Build history of the part. All positions in model axes, mm. Coordinates: 2 decimals unless noted, no trailing zeros. Loops run counter-clockwise (first coordinate to the right, second up) from the corner with the lowest first, then second, coordinate; pieces in that order, holes last. Notation, with made-up numbers: M 36.25,61.5 L 44.25,61.5 A32 cw 44.25,97.5 Z; hole C 8,33 d1. An arc over 180 degrees is marked long. Write each question's results on one line, items separated by ' | '. Start each with the question number.
from build123d import *

# Parameters (mm, degrees)
PRISM002_DEPTH           = 2.6
PRISM002_PLACEMENT_ANGLE = 45
ARRAY_COUNT              = 4
CYLINDER003_R            = 5.25
CYLINDER003_DEPTH        = 36
CYLINDER003_ROLL_ANGLE   = 90
SKETCH011_R              = 29
PAD006_DEPTH             = 16
SKETCH_R                 = 27.4
POCKET_DEPTH             = 1
SKETCH012_R              = 1.6
POCKET003_DEPTH          = 13
SKETCH013_W              = 16
SKETCH013_H              = 4
PAD_DEPTH                = 4
POCKET004_DEPTH          = 24
CHAMFER_SIZE             = 1


with BuildPart() as array:
    # Prism002 → Prism002 (new body)
    with BuildSketch(Plane.XY):
        Polygon((3.1, 0), (1.55, 2.684679), (-1.55, 2.684679), (-3.1, 0), (-1.55, -2.684679), (1.55, -2.684679), align=None)
    extrude(amount=PRISM002_DEPTH)


with BuildPart() as array_1:
    # Prism002 placement: moved
    add(array.part.moved(Location((-15.5563, 15.5563, 12.4))).rotate(Axis((-15.5563, 15.5563, 12.4), (0, 0, 1)), PRISM002_PLACEMENT_ANGLE))

    # Array: Array ×4 about axis
    array_axis = Axis((0, 0, 0), (0, 0, 1))


with BuildPart() as array_2:
    add(array_1.part)
    for i in range(1, ARRAY_COUNT):
        add(array_1.part.rotate(array_axis, i * 360 / ARRAY_COUNT))


with BuildPart() as laser_pointer:
    # Cylinder003 → Cylinder003 (new body)
    with BuildSketch(Plane.XY):
        Circle(CYLINDER003_R)
    extrude(amount=CYLINDER003_DEPTH)


with BuildPart() as laser_pointer_1:
    # Cylinder003 roll: moved
    add(laser_pointer.part.rotate(Axis((0, 0, 0), (1, 0, 0)), CYLINDER003_ROLL_ANGLE))


with BuildPart() as laser_pointer_2:
    # Cylinder003 placement: moved
    add(laser_pointer_1.part.moved(Location((0, 30, 8.5))))


with BuildPart() as laser_enclosure:
    # Sketch011 → Pad006 (new body)
    with BuildSketch(Plane.XY):
        Circle(SKETCH011_R)
    extrude(amount=PAD006_DEPTH)

    # Sketch → Pocket (cut)
    with BuildSketch(Plane.XY.offset(16)):
        Circle(SKETCH_R)
    extrude(amount=-POCKET_DEPTH, mode=Mode.SUBTRACT)

    # Sketch012 → Pocket003 (cut)
    with BuildSketch(Plane.XY.offset(15)):
        with Locations((-15.556349, 15.556349)):
            Circle(SKETCH012_R)
        with Locations((-15.556349, -15.556349)):
            Circle(SKETCH012_R)
        with Locations((15.556349, -15.556349)):
            Circle(SKETCH012_R)
        with Locations((15.556349, 15.556349)):
            Circle(SKETCH012_R)
        with BuildLine():
            ThreePointArc((-15.072779, -21.917375), (0, -26.6), (15.072779, -21.917375))
            Line((15.072779, -21.917375), (12.149548, -18.340897))
            ThreePointArc((18.340897, -12.149548), (12.445079, -12.445079), (12.149548, -18.340897))
            Line((21.91738, -15.072773), (18.340897, -12.149548))
            ThreePointArc((21.91738, -15.072773), (26.6, 4e-06), (21.917375, 15.072779))
            Line((21.917375, 15.072779), (18.340897, 12.149548))
            ThreePointArc((12.149548, 18.340897), (12.445079, 12.445079), (18.340897, 12.149548))
            Line((15.072779, 21.917375), (12.149548, 18.340897))
            ThreePointArc((15.072779, 21.917375), (0, 26.6), (-15.072779, 21.917375))
            Line((-15.072779, 21.917375), (-12.149548, 18.340897))
            ThreePointArc((-18.340897, 12.149548), (-12.445079, 12.445079), (-12.149548, 18.340897))
            Line((-21.917375, 15.072779), (-18.340897, 12.149548))
            ThreePointArc((-21.917375, 15.072779), (-26.6, 0), (-21.917375, -15.072779))
            Line((-21.917375, -15.072779), (-18.340897, -12.149548))
            ThreePointArc((-12.149548, -18.340897), (-12.445079, -12.445079), (-18.340897, -12.149548))
            Line((-15.072779, -21.917375), (-12.149548, -18.340897))
        make_face()
    extrude(amount=-POCKET003_DEPTH, mode=Mode.SUBTRACT)

    # Sketch013 → Pad (new body)
    with BuildSketch(Plane.XY.offset(2)):
        with Locations((0, 14)):
            Rectangle(SKETCH013_W, SKETCH013_H)
        with Locations((0, -4)):
            Rectangle(SKETCH013_W, SKETCH013_H)
    extrude(amount=PAD_DEPTH)

    # Sketch014 → Pocket004 (cut)
    with BuildSketch(Plane.XZ.offset(6)):
        Polygon((5.985281, 6), (1.985281, 2), (-1.985281, 2), (-5.985281, 6), align=None)
    extrude(amount=-POCKET004_DEPTH, mode=Mode.SUBTRACT)

    # Cut: cut Laser pointer
    add(laser_pointer_2.part, mode=Mode.SUBTRACT)

    # Cut001: cut Array
    add(array_2.part, mode=Mode.SUBTRACT)

    # Chamfer
    chamfer_edges = [laser_enclosure.edges().sort_by_distance(p)[0] for p in [
        (-29, 0, 0),
    ]]
    chamfer(chamfer_edges, length=CHAMFER_SIZE)


solid = laser_enclosure.part
1. Band-saw the part on C-C, the plane z = 6.75. List the corners of the cut face in (x, y), plus the area to 3 significant figures.
2. Band-saw the part on A-A, the plane x = 0. List the corners of the cut face in (y, z), plus the area to 3 significant figures.
3. Mould opens along X. For faces 1 (the cylindrical face through (13.958, -15.486, 7.273)), 2 (the flat face through (0, 0, 0)), 3 (the cylindrical face through (13.38, -25.73, 8.4)) say: +X half, -X half, draft (parallel to the pull), parting line (faces both ways), or undercut.
4. Wall check: line 1 along Y through (x, z) = (-14.5, 2.5); line 2 along Z through (x, y) = (0, 27.6); line 3 along Y through (x, z) = (-12.5, 9). Give the ranges that are in metal, low to high.
5. Pin check, flat tips, straight feed: pin 1 (2 mm diameter, centred on x = 6.5, z = 5.5, fed in from +Y); pin 2 (3 mm diameter, centred on x = 15.56, y = -15.56, fed in from +Z); pin 3 (3 mm diameter, centred on x = 8, z = 5, fed in from +Y). Stop position of each tip, or through.
6. Band-saw the part on B-B, the plane z = 11. List the corners of the cut face in (x, y).
Checked values:
1) outline: M -21.92,-15.07 A26.6 cw -21.92,15.07 L -18.34,12.15 A4.4 ccw -12.15,18.34 L -15.07,21.92 A26.6 cw -4.95,26.14 L -4.95,28.57 A29 ccw long 4.95,28.57 L 4.95,26.14 A26.6 cw 15.07,21.92 L 12.15,18.34 A4.4 ccw 18.34,12.15 L 21.92,15.07 A26.6 cw 21.92,-15.07 L 18.34,-12.15 A4.4 ccw 12.15,-18.34 L 15.07,-21.92 A26.6 cw -15.07,-21.92 L -12.15,-18.34 A4.4 ccw -18.34,-12.15 Z; hole C -15.56,-15.56 d3.2; hole C -15.56,15.56 d3.2; hole C 15.56,-15.56 d3.2; hole C 15.56,15.56 d3.2 | area: 650 mm²
2) outline: M -29,1 L -28,0 L 28,0 L 29,1 L 29,3.25 L 26.6,3.25 L 26.6,2 L -26.6,2 L -26.6,15 L -27.4,15 L -27.4,16 L -29,16 Z; M 26.6,13.75 L 29,13.75 L 29,16 L 27.4,16 L 27.4,15 L 26.6,15 Z | area: 155 mm²
3) face 1: undercut | face 2: draft | face 3: parting line
4) line 1: -25.11 to -22.3, -21.22 to -16.76, -14.35 to -11.29, 11.29 to 14.35, 16.76 to 21.22, 22.3 to 25.11 | line 2: 0 to 3.25, 13.75 to 16 | line 3: -26.17 to -23.48, -18.77 to -12.39, 12.39 to 18.77, 23.48 to 26.17
5) pin 1: y = 28.47 | pin 2: z = 2 | pin 3: y = 28.26
6) outline: M -21.92,-15.07 A26.6 cw -21.92,15.07 L -18.34,12.15 A4.4 ccw -12.15,18.34 L -15.07,21.92 A26.6 cw -4.62,26.2 L -4.62,28.63 A29 ccw long 4.62,28.63 L 4.62,26.2 A26.6 cw 15.07,21.92 L 12.15,18.34 A4.4 ccw 18.34,12.15 L 21.92,15.07 A26.6 cw 21.92,-15.07 L 18.34,-12.15 A4.4 ccw 12.15,-18.34 L 15.07,-21.92 A26.6 cw -15.07,-21.92 L -12.15,-18.34 A4.4 ccw -18.34,-12.15 Z; hole C -15.56,-15.56 d3.2; hole C -15.56,15.56 d3.2; hole C 15.56,-15.56 d3.2; hole C 15.56,15.56 d3.2
